Autodesk Inventor part; units mm, degrees
ref_plane "YZ Plane" through (0, 0, 0) normal (1, 0, 0) x (0, 1, 0)
ref_plane "XZ Plane" through (0, 0, 0) normal (0, 1, 0) x (-1, 0, 0)
ref_plane "XY Plane" through (0, 0, 0) normal (0, 0, 1) x (1, 0, 0)
sketch "Sketch1" plane through (0, 0, 0) normal (0, 0, 1) x (1, 0, 0)
  line L0 (-28.5, -28.5) -> (28.5, -28.5)
  line L1 (28.5, -28.5) -> (28.5, 28.5)
  line L2 (28.5, 28.5) -> (-28.5, 28.5)
  line L3 (-28.5, 28.5) -> (-28.5, -28.5)
  line L4 (-28.5, -28.5) -> (28.5, 28.5) construction
  line L5 (28.5, -28.5) -> (-28.5, 28.5) construction
  point P0 (0, 0)
  dimension "d0" = 57
  dimension "d1" = 57
extrude "Extrusion1" add sketch "Sketch1" against normal blind 2.921
sketch "Sketch4" plane through (0, 0, 0) normal (0, 0, 1) x (1, 0, 0)
  line L0 (28.5, -25.5) -> (9.5, -25.5)
  line L1 (9.5, -25.5) -> (9.5, -28.5)
  line L2 (9.5, -28.5) -> (28.5, -28.5)
  line L3 (28.5, -28.5) -> (28.5, -25.5)
  line L4 (-28.5, -28.5) -> (-9.5, -28.5)
  line L5 (-9.5, -28.5) -> (-9.5, -25.5)
  line L6 (-9.5, -25.5) -> (-28.5, -25.5)
  line L7 (-28.5, -25.5) -> (-28.5, -28.5)
  line L8 (28.5, -28.5) -> (28.5, 28.5)
  line L9 (28.5, 28.5) -> (-28.5, 28.5)
  line L10 (-28.5, 28.5) -> (-28.5, -28.5)
  line L11 (-28.5, 15.5) -> (-25.5, 15.5)
  line L12 (-25.5, 15.5) -> (-25.5, -3.5)
  line L13 (-25.5, -3.5) -> (-28.5, -3.5)
  line L14 (-28.5, -3.5) -> (-28.5, 15.5)
  line L15 (28.5, 15.5) -> (25.5, 15.5)
  line L16 (25.5, 15.5) -> (25.5, -3.5)
  line L17 (25.5, -3.5) -> (28.5, -3.5)
  line L18 (28.5, -3.5) -> (28.5, 15.5)
  line L19 (-9.5, 28.5) -> (9.5, 28.5)
  line L20 (9.5, 28.5) -> (9.5, 25.5)
  line L21 (9.5, 25.5) -> (-9.5, 25.5)
  line L22 (-9.5, 25.5) -> (-9.5, 28.5)
  line L23 (-28.5, -28.5) -> (28.5, -28.5)
  line L24 (25.5, -3.5) -> (25.5, -28.5)
  line L25 (25.5, 15.5) -> (25.5, 28.5)
  point P0 (0, 0)
  dimension "d12" = 19
  dimension "d13" = 3
  dimension "d16" = 3
  dimension "d37" = 9.5
  dimension "d38" = 19
  dimension "d39" = 9.5
  dimension "d40" = 3
  dimension "d41" = 3
  dimension "d42" = 19
  dimension "d43" = 19
  dimension "d44" = 3
  dimension "d45" = 19
  dimension "d46" = 19
  dimension "d50" = 25
  dimension "d51" = 25
  dimension "d52" = 19
  dimension "d53" = 57
  dimension "d54" = 57
extrude "Extrusion5" cut sketch "Sketch4" against normal blind 25.4 contours L3 L2 L24 L0 | L0 L24 L17 L8 | L24 L2 L1 L0 | L15 L25 L9 L8 | L4 L7 L6 L5 | L20 L21 L22 L9 | L10 L11 L12 L13
hole "Hole1" at (0, 0, 0) direction (0, 0, -1) diameter 25.4 end through all
equation "\"d1\" = d0"
equation "\"d12\" = d38"
equation "\"d13\" = d16"
equation "\"d16\" = d44"
equation "\"d38\" = d45"
equation "\"d40\" = d44"
equation "\"d41\" = d16"
equation "\"d42\" = d45"
equation "\"d43\" = d42"
equation "\"d46\" = d45"
equation "\"d51\" = d50"
equation "\"d19\" = 0.5 * d0"
equation "\"d48\" = 0.5 * d0"
properties part number "Side B"
Can you work these out from the model? Positions are in its coordinate system, mm. A direction names the side the tool comes from. Give positions to 0.01 mm unless a question says otherwise; leave off trailing zeros. Order: outer loops, then holes, each group sorted by start corner. A loop starts at its lowest first (then second) coordinate and runs counter-clockwise, first axis right, second up. Notation, with made-up numbers: M -36,30.25 L -7,30.25 A19 ccw -7,61.25 Z; hole C 70,-5.75 d11. An arc over 180 degrees is marked long. One line per item, written item: value.
Item 1: For faces 1 (the face through (25.5, 22, -1)), 2 (the face through (0, 25.5, -1)), 3 (the face through (12.4, 2.75, -1.48)), 4 (the face through (-27, 15.5, -1)), 5 (the face through (25.5, -14, -1)), which set-ups out of +Z, -Z, +X, -X, +Y, -Y let a thin tool reach every point of the face, with its end or its side?
Verdict:
face 1: +Z, -Z, +X, +Y
face 2: +Z, -Z, +Y
face 3: +Z, -Z
face 4: +Z, -Z, -X
face 5: +Z, -Z, +X, -Y
Item 2: If we section it at A-A on y = 0: Write out the boundary of the cut face in (x, z).
Verdict:
outline: M -25.5,-2.92 L -12.7,-2.92 L -12.7,0 L -25.5,0 Z; M 12.7,-2.92 L 28.5,-2.92 L 28.5,0 L 12.7,0 Z
Item 3: Please list where these lines run through material, in increasing order: line 1 (Y direction, x = 0, z = -1.75); line 2 (X direction, y = 0, z = -1.45); line 3 (Y direction, x = -7, z = -2.6).
Verdict:
line 1: -28.5 to -12.7, 12.7 to 25.5
line 2: -25.5 to -12.7, 12.7 to 28.5
line 3: -28.5 to -10.6, 10.6 to 25.5
Item 4: If we mould it in two halves opening along X, with no side actions, what happens to faces 6 (the face through (0, -28.5, -1)), 7 (the face through (9.5, -27, -1)), 8 (the face through (-9.5, 27, -1)), 9 (the face through (-9.5, -27, -1))? For each: pulls with the +X half, pulls with the -X half, needs draft (parallel to the pull), parting line crosses it, or undercut.
Verdict:
face 6: needs draft
face 7: pulls with the +X half
face 8: undercut
face 9: pulls with the -X half
Item 5: For pin 1 (0.9 mm diameter, centred on y = -27, z = -1.5, fed in from +X); pin 2 (1.5 mm diameter, centred on x = 20, z = -1.5, fed in from -Y); pin 3 (0.9 mm diameter, centred on y = 27, z = -2, fed in from +X), each with a flat end and sliding along its axis, tell me the tip position at first contact or that it passes through.
Verdict:
pin 1: x = 9.5
pin 2: y = -25.5
pin 3: x = 25.5
Item 6: If we section it at B-B on x = 0: Write out the boundary of the cut face in (y, z), and give its area (3 significant figures).
Verdict:
outline: M -28.5,-2.92 L -12.7,-2.92 L -12.7,0 L -28.5,0 Z; M 12.7,-2.92 L 25.5,-2.92 L 25.5,0 L 12.7,0 Z
area: 83.5 mm2
Item 7: If we section it at D-D on y = -20: Write out the boundary of the cut face in (x, z), and give its area (3 significant figures).
Verdict:
outline: M -28.5,-2.92 L 25.5,-2.92 L 25.5,0 L -28.5,0 Z
area: 158 mm2
Item 8: If we section it at C-C on z = -1.55: Write out the boundary of the cut face in (x, y).
Verdict:
outline: M -28.5,-25.5 L -9.5,-25.5 L -9.5,-28.5 L 9.5,-28.5 L 9.5,-25.5 L 25.5,-25.5 L 25.5,-3.5 L 28.5,-3.5 L 28.5,15.5 L 25.5,15.5 L 25.5,28.5 L 9.5,28.5 L 9.5,25.5 L -9.5,25.5 L -9.5,28.5 L -28.5,28.5 L -28.5,15.5 L -25.5,15.5 L -25.5,-3.5 L -28.5,-3.5 Z; hole C 0,0 d25.4
